```python
from build123d import *

# Parameters (mm, degrees)
SKETCH_1_R          = 16
SKETCH_1_R_2        = 2.0000000000000004
SKETCH_1_R_3        = 2.0000000000000013
SKETCH_1_R_4        = 1.9999999999999996
EXTRUDE_1_DEPTH     = 3
EXTRUDE_START       = 12
EXTRUDE_2_DEPTH     = 12
SKETCH_4_R          = 1.5000000000000009
SKETCH_4_R_2        = 1.5000000000024705
SKETCH_4_R_3        = 1.5000000000036489
CUT_EXTRUDE_1_DEPTH = 71.79051465905462
FILLET_1_R          = 2
FILLET_2_R          = 3


with BuildPart() as part:
    # 草图1 → 凸台-拉伸1 (new body)
    with BuildSketch(Plane.XY):
        with BuildLine():
            Line((5.623776358596461, 24.359251619630925), (11.247552717192923, 48.71850323926185))
            ThreePointArc((11.247552717192923, 48.71850323926185), (-3.7441e-13, 50.000000000000014), (-11.247552717193646, 48.71850323926167))
            Line((-11.247552717193646, 48.71850323926167), (-5.623776358596823, 24.359251619630832))
            ThreePointArc((-5.623776358596823, 24.359251619630832), (-21.650635094611058, 12.499999999999835), (-23.90761889907584, -7.309292618068593))
            Line((-23.90761889907584, -7.309292618068593), (-47.81523779815182, -14.61858523613672))
            ThreePointArc((-47.81523779815182, -14.61858523613672), (-43.30127018922199, -24.999999999999925), (-36.56768508095856, -34.099918003124884))
            Line((-36.56768508095856, -34.099918003124884), (-18.28384254047911, -17.04995900156262))
            ThreePointArc((-18.28384254047911, -17.04995900156262), (2.0137e-13, -24.999999999999996), (18.283842540479387, -17.04995900156234))
            Line((18.283842540479387, -17.04995900156234), (36.56768508095862, -34.09991800312487))
            ThreePointArc((36.56768508095862, -34.09991800312487), (43.30127018922202, -24.999999999999897), (47.815237798151834, -14.618585236136676))
            Line((47.815237798151834, -14.618585236136676), (23.907618899075946, -7.309292618068216))
            ThreePointArc((23.907618899075946, -7.309292618068216), (21.650635094610866, 12.500000000000162), (5.623776358596461, 24.359251619630925))
        make_face()
        Circle(SKETCH_1_R, mode=Mode.SUBTRACT)
        with Locations((1.302e-14, 20)):
            Circle(SKETCH_1_R_2, mode=Mode.SUBTRACT)
        with Locations((17.320508075688725, -10.000000000000092)):
            Circle(SKETCH_1_R_3, mode=Mode.SUBTRACT)
        with Locations((-17.320508075688874, -9.999999999999826)):
            Circle(SKETCH_1_R_4, mode=Mode.SUBTRACT)
    extrude(amount=EXTRUDE_1_DEPTH)

    # 草图3 → 凸台-拉伸2 (add)
    with BuildSketch(Plane(origin=(0, 0, 0), x_dir=(-1, 0, 0), z_dir=(0, 0, -1)).offset(EXTRUDE_START)):
        with BuildLine():
            Line((-11.247552717192923, 48.71850323926185), (-9.222993228098195, 39.949172656194705))
            ThreePointArc((-9.222993228098195, 39.949172656194705), (3.0294e-13, 41), (9.22299322809879, 39.94917265619457))
            Line((9.22299322809879, 39.94917265619457), (11.247552717193646, 48.71850323926167))
            ThreePointArc((11.247552717193646, 48.71850323926167), (3.8054e-13, 50), (-11.247552717192923, 48.71850323926185))
        make_face()
        with BuildLine():
            Line((47.815237798151635, -14.618585236137392), (39.20849499448435, -11.987239893632658))
            ThreePointArc((39.20849499448435, -11.987239893632658), (35.507041555161756, -20.500000000000437), (29.98550176638565, -27.96193276256283))
            Line((29.98550176638565, -27.96193276256283), (36.56768508095811, -34.099918003125396))
            ThreePointArc((36.56768508095811, -34.099918003125396), (43.30127018922164, -25.00000000000053), (47.815237798151635, -14.618585236137392))
        make_face()
        with BuildLine():
            Line((-36.56768508095907, -34.09991800312435), (-29.98550176638619, -27.96193276256223))
            ThreePointArc((-29.98550176638619, -27.96193276256223), (-35.50704155516215, -20.499999999999734), (-39.20849499448456, -11.987239893631878))
            Line((-39.20849499448456, -11.987239893631878), (-47.815237798152026, -14.618585236136003))
            ThreePointArc((-47.815237798152026, -14.618585236136003), (-43.30127018922234, -24.999999999999286), (-36.56768508095907, -34.09991800312435))
        make_face()
    extrude(amount=-EXTRUDE_2_DEPTH)

    # 草图4 → 切除-拉伸1 (cut, through all)
    with BuildSketch(Plane.XY.offset(3)):
        with Locations((0, 45)):
            Circle(SKETCH_4_R)
        with Locations((38.97114317030261, -22.499999999998334)):
            Circle(SKETCH_4_R_2)
        with Locations((-38.97114317029686, -22.500000000001673)):
            Circle(SKETCH_4_R_3)
    extrude(amount=-CUT_EXTRUDE_1_DEPTH, mode=Mode.SUBTRACT)

    # 圆角1
    fillet_1_edges = [part.edges().sort_by_distance(p)[0] for p in [
        (5.623776358596462, 24.359251619630925, 1.5),
        (23.907618899075946, -7.309292618068216, 1.5),
        (18.283842540479387, -17.049959001562343, 1.5),
        (-18.28384254047911, -17.04995900156262, 1.5),
        (-23.90761889907584, -7.309292618068593, 1.5),
        (-5.623776358596823, 24.359251619630832, 1.5),
    ]]
    fillet(fillet_1_edges, radius=FILLET_1_R)

    # 圆角2
    fillet_2_edges = [part.edges().sort_by_distance(p)[0] for p in [
        (11.24755271719292, 48.71850323926185, -4.5),
        (47.81523779815193, -14.61858523613634, -4.5),
        (36.567685080958846, -34.099918003124614, -4.5),
        (-36.56768508095834, -34.09991800312514, -4.5),
        (-47.81523779815173, -14.618585236137056, -4.5),
        (-11.247552717193646, 48.71850323926167, -4.5),
        (-39.208494994484354, -11.987239893632658, -6),
        (-29.985501766385653, -27.96193276256283, -6),
        (9.222993228098195, 39.949172656194705, -6),
        (-9.222993228098792, 39.94917265619457, -6),
        (29.98550176638619, -27.96193276256223, -6),
        (39.20849499448456, -11.987239893631878, -6),
    ]]
    fillet(fillet_2_edges, radius=FILLET_2_R)


solid = part.part
```
Could you check a few things on this model? Use its own coordinates, in mm. A direction names the side the tool comes from. Coordinates: 2 decimals unless noted, no trailing zeros. Loops run counter-clockwise (first coordinate to the right, second up) from the corner with the lowest first, then second, coordinate; pieces in that order, holes last.
1) Please list where these lines run through material, in increasing order: line 1 along X through (y, z) = (-22, -3); line 2 along Z through (x, y) = (23.5, 7); line 3 along X through (y, z) = (-28, -5.5).
Reported:
line 1: x = -44.9 to -40.39, -37.56 to -34.6, 34.6 to 37.56, 40.39 to 44.9
line 2: z = 0 to 3
line 3: x = -41.42 to -31.16, 31.16 to 41.42
2) Will these pins go through, and if not, where does the flat tip stop? pin 1 Ø1.5 at (x, z) = (2, -8) entering from +Y; pin 2 Ø6.5 at (x, y) = (17.32, -10) entering from -Z; pin 3 Ø8 at (x, z) = (-7, -4.5) entering from -Y.
Reported:
pin 1: stops at y = 49.98
pin 2: stops at z = 0
pin 3: stops at y = 40.45
3) Imagine slicing it at A-A (x = 0). List the corners of the cut face in (y, z) for me.
Reported:
outline: (-25, 0) - (-16, 0) - (-16, 3) - (-25, 3) - close; (16, 0) - (18, 0) - (18, 3) - (16, 3) - close; (22, 0) - (41, 0) - (41, -12) - (43.5, -12) - (43.5, 3) - (22, 3) - close; (46.5, -12) - (50, -12) - (50, 3) - (46.5, 3) - close
4) Imagine slicing it at D-D (y = -10). List the corners of the cut face in (x, z) for me.
Reported:
outline: (-32.71, 0) - (-19.32, 0) - (-19.32, 3) - (-32.71, 3) - close; (-15.32, 0) - (-12.49, 0) - (-12.49, 3) - (-15.32, 3) - close; (12.49, 0) - (15.32, 0) - (15.32, 3) - (12.49, 3) - close; (19.32, 0) - (32.71, 0) - (32.71, 3) - (19.32, 3) - close
5) Thinking about a two-plate mould opening in X: for faces 6 (the face through (6.26, 24.81, 1.52)), 7 (the face through (-8.96, 38.81, 0.46)), 8 (the face through (35.46, -20.58, -6.08)), which applies, released by +X, released by -X, zero draft, split by the parting line, or undercut?
Reported:
face 6: released by +X
face 7: released by -X
face 8: undercut
6) Which directions (+Z, -Z, +X, -X, +Y, -Y) give clear straight access to the entire face, cutting with the end or side of a thin tool? Please do faces 1 (the face through (-35.552, -20.421, -6.084)), 2 (the face through (-29.738, -27.731, 0.465)), 3 (the face through (31.16, -27.98, -5.92)), 4 (the face through (9.147, 39.619, 0.465)), 5 (the face through (14, 9, 3)).
Reported:
face 1: -Z, +Y
face 2: +Z, -Z, -Y
face 3: -Z
face 4: +Z, -Z, +X
face 5: +Z, +X, -X, +Y, -Y
7) Imagine slicing it at C-C (z = -3.75). List the corners of the cut face in (x, y) for me, and give its area (3 significant figures).
Reported:
outline: (-46.78, -17.64) arc R50 ccw to (-38.67, -31.7) arc R3 ccw to (-34.3, -31.99) - (-32.1, -29.94) arc R3 ccw to (-31.82, -25.85) arc R41 cw to (-38.3, -14.63) arc R3 ccw to (-41.98, -12.83) - (-44.85, -13.71) arc R3 ccw to start; (-10.55, 45.7) - (-9.87, 42.77) arc R3 ccw to (-6.48, 40.49) arc R41 cw to (6.48, 40.49) arc R3 ccw to (9.87, 42.77) - (10.55, 45.7) arc R3 ccw to (8.11, 49.34) arc R50 ccw to (-8.11, 49.34) arc R3 ccw to start; (31.82, -25.85) arc R3 ccw to (32.1, -29.94) - (34.3, -31.99) arc R3 ccw to (38.67, -31.7) arc R50 ccw to (46.78, -17.64) arc R3 ccw to (44.85, -13.71) - (41.98, -12.83) arc R3 ccw to (38.3, -14.63) arc R41 cw to start; hole circle Ø3 at (-38.97, -22.5); hole circle Ø3 at (0, 45); hole circle Ø3 at (38.97, -22.5)
area: 513 mm2
8) Imagine slicing it at B-B (y = 0). List the corners of the cut face in (x, z) for me, and give its area (3 significant figures).
Reported:
outline: (-25, 0) - (-16, 0) - (-16, 3) - (-25, 3) - close; (16, 0) - (25, 0) - (25, 3) - (16, 3) - close
area: 54.0 mm2
